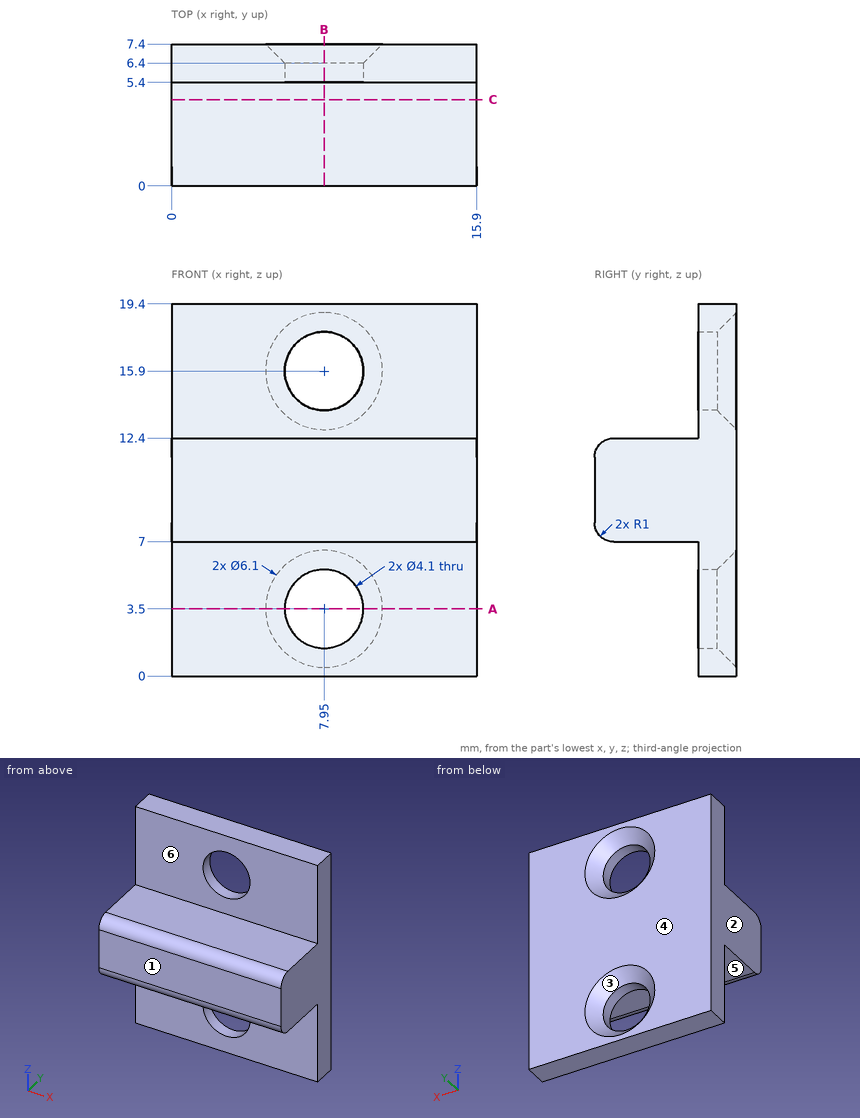
Source: three-view drawing plus pictorial views. Frame: mm from the lowest corner of the part. A direction names the side the tool comes from. Round coordinates to 2 decimals unless told otherwise and drop trailing zeros. Loops run counter-clockwise (first coordinate to the right, second up) from the corner with the lowest first, then second, coordinate; pieces in that order, holes last.
Q1. Section C-C, the plane y = 4.5. Return loops of the section in (x, z).
Q2. Section A-A, the plane z = 3.5. Return loops of the section in (x, y).
Q3. Access query for the marked faces 4, 5 and 6. Directions: +Z, -Z, +X, -X, +Y, -Y. A direction counts if a zero-diameter tool reaches every point of the face in a straight line with its end or side. Return the directions, or none.
Q4. Mould query, pull axis X, two halves, no side actions, for the marked faces 1, 2 and 3. Classes: pulls with the +X half, pulls with the -X half, needs draft (parallel to the pull), parting line crosses it, or undercut.
Q5. Ray query, line 1 (X direction, y = 6.2, z = 3.5); line 2 (Z direction, x = 8, y = 7); line 3 (Y direction, x = 4.5, z = 13.5). Return the intervals inside material, ascending.
Q6. First-contact query: P1, Ø4.5, axis at x = 7.95, z = 15.9, coming from the +Y side; P2, Ø7.5, axis at x = 8, z = 16.5, coming from the -Y side; P3, Ø2, axis at x = 7.5, y = 2, coming from the +Z side. Flat tips, straight axial feed; report the tip coordinate or a pass-through.
Q7. Section B-B, the plane x = 7.95. Return loops of the section in (y, z).
Solutions:
1. outline: (0, 7) - (15.9, 7) - (15.9, 12.4) - (0, 12.4) - close
2. outline: (0, 5.4) - (5.9, 5.4) - (5.9, 6.4) - (4.9, 7.4) - (0, 7.4) - close; (10, 5.4) - (15.9, 5.4) - (15.9, 7.4) - (11, 7.4) - (10, 6.4) - close
3. face 4: +Z, -Z, +X, -X, +Y
3. face 5: -Z, +X, -X, -Y
3. face 6: +Z, +X, -X, -Y
4. face 1: needs draft
4. face 2: pulls with the -X half
4. face 3: undercut
5. line 1: x = 0 to 5.9, 10 to 15.9
5. line 2: z = 0 to 0.85, 6.15 to 13.25, 18.55 to 19.4
5. line 3: y = 5.4 to 7.4
6. P1: stops at y = 6.6
6. P2: stops at y = 5.4
6. P3: stops at z = 12.4
7. outline: (0, 8) arc R1 ccw to (1, 7) - (5.4, 7) - (5.4, 5.55) - (6.4, 5.55) - (7.4, 6.55) - (7.4, 12.85) - (6.4, 13.85) - (5.4, 13.85) - (5.4, 12.4) - (1, 12.4) arc R1 ccw to (0, 11.4) - close; (5.4, 0) - (7.4, 0) - (7.4, 0.45) - (6.4, 1.45) - (5.4, 1.45) - close; (5.4, 17.95) - (6.4, 17.95) - (7.4, 18.95) - (7.4, 19.4) - (5.4, 19.4) - close
